Work out the finished part from the listing and answer in its coordinate system (mm). A direction names the side the tool comes from. Round coordinates to 2 decimals unless told otherwise and drop trailing zeros. Write each loop counter-clockwise with the first axis right and the second up, starting at its lowest first coordinate (ties: lowest second). Pieces come first, ordered by that corner, then holes. Notation, with made-up numbers: M 77.25,-8 L 86.25,-8 A18 cw 86.25,6 Z; hole C -28,41.5 d3. An arc over 180 degrees is marked long. One line per item, written item: value. Start each with the question number.
Q1. Consider probe 1 along Y at (x, z) = (24, 0.5); probe 2 along Z at (x, y) = (20, 40.2); probe 3 along Y at (x, z) = (15.5, 2.75). Determine where each line is inside the solid, lowest interval first.
Q2. A tool of negligible diameter and unlimited length cuts with its end or side. For faces 4 (the flat face through (28, 18, 0)), 5 (the cylindrical face through (20.737, 40.918, 6.676)), 6 (the flat face through (3, 42, 10.15)), from which of +Z, -Z, +X, -X, +Y, -Y can it reach the whole face along a straight path? Write none if from no direction.
Q3. Find section B-B (z = -2.5). Write down the section's boundary in (x, y), and give its area (3 significant figures).
Q4. Given pin 1 Ø4.5 at (y, z) = (12, -2.5) entering from -X; pin 2 Ø8 at (x, y) = (18.5, 1.5) entering from -Z; pin 3 Ø1 at (y, z) = (23, 7) entering from -X, each flat-ended and moving along its own axis, determine where each tip first touches the part or whether it passes through.
Q5. Find section C-C (z = 8.5). Write down the section's boundary in (x, y), and give its area (3 significant figures).
Q6. The mould has two halves that part along X. Classify faces 1 (the flat face through (16.584, 42.91, 9.576)), 2 (the flat face through (26.3, 22.44, -1.5)), 3 (the cylindrical face through (9.7, -2.03, 8.95)): released by +X, released by -X, zero draft, split by the parting line, or undercut.
Q7. Find section D-D (x = 20). Write down the section's boundary in (y, z).
Q8. Find section A-A (x = 15.25). Write down the section's boundary in (y, z).
from build123d import *

# Parameters (mm, degrees)
EXTRUDE_1_DEPTH     = 12
SKETCH_2_R          = 4
CUT_EXTRUDE_1_DEPTH = 4
CUT_EXTRUDE_2_DEPTH = 4
SKETCH_4_R          = 1
CUT_EXTRUDE_3_DEPTH = 1.4
CUT_EXTRUDE_4_DEPTH = 4
EXTRUDE_START       = 6
SKETCH_5_W          = 6
SKETCH_5_H          = 5
SKETCH_5_R          = 1
EXTRUDE_2_DEPTH     = 4
EXTRUDE_START_2     = -6
SKETCH_5_2_W        = 6
SKETCH_5_2_H        = 5
SKETCH_5_2_R        = 1
EXTRUDE_3_DEPTH     = 4
FILLET_1_R          = 2


with BuildPart() as part:
    # 草图1 → 凸台-拉伸1 (new body)
    with BuildSketch(Plane.XY):
        Polygon((0, 0), (26, 0), (26, 39.6), (0, 39.6), (0, 43.6), (30, 43.6), (30, -4), (0, -4), align=None)
    extrude(amount=EXTRUDE_1_DEPTH)

    # 草图2 → 切除-拉伸1 (cut)
    with BuildSketch(Plane.XZ.offset(4)):
        with Locations(Location((7, 6, 0), (0, 0, 270))):
            Circle(SKETCH_2_R)
    extrude(amount=-CUT_EXTRUDE_1_DEPTH, mode=Mode.SUBTRACT)

    # 草图3 → 切除-拉伸2 (cut)
    with BuildSketch(Plane(origin=(0, 43.6, 0), x_dir=(1, 0, 0), z_dir=(0, 1, 0))):
        with BuildLine():
            Line((0, -1.85), (0, -10.15))
            Line((0, -10.15), (7, -10.15))
            ThreePointArc((7, -10.15), (11.15, -6), (7, -1.85))
            Line((7, -1.85), (0, -1.85))
        make_face()
    extrude(amount=-CUT_EXTRUDE_2_DEPTH, mode=Mode.SUBTRACT)

    # 草图4 → 切除-拉伸3 (cut)
    with BuildSketch(Plane(origin=(0, 43.6, 0), x_dir=(1, 0, 0), z_dir=(0, 1, 0))):
        with BuildLine():
            ThreePointArc((7.251184211, -1.857608602), (11.15, -6), (7.251184211, -10.142391398))
            Line((7.251184211, -10.142391398), (26.181578947, -8.994499806))
            ThreePointArc((26.181578947, -8.994499806), (29, -6), (26.181578947, -3.005500194))
            Line((26.181578947, -3.005500194), (7.251184211, -1.857608602))
        make_face()
        with Locations(Location((23, -6, 0), (0, 0, 270))):
            Circle(SKETCH_4_R, mode=Mode.SUBTRACT)
        with Locations(Location((20, -6, 0), (0, 0, 270))):
            Circle(SKETCH_4_R, mode=Mode.SUBTRACT)
        with Locations(Location((17, -6, 0), (0, 0, 270))):
            Circle(SKETCH_4_R, mode=Mode.SUBTRACT)
    extrude(amount=-CUT_EXTRUDE_3_DEPTH, mode=Mode.SUBTRACT)

    # 草图4<3> → 切除-拉伸4 (cut)
    with BuildSketch(Plane(origin=(0, 43.6, 0), x_dir=(1, 0, 0), z_dir=(0, 1, 0))):
        with BuildLine():
            ThreePointArc((23, -6), (23.041960108, -6.5), (23.166666667, -6.986013297))
            ThreePointArc((23.166666667, -6.986013297), (23.763762616, -6.645497224), (24, -6))
            Line((24, -6), (23, -6))
        make_face()
        with BuildLine():
            ThreePointArc((22, -6), (22.354502776, -6.763762616), (23.166666667, -6.986013297))
            ThreePointArc((23.166666667, -6.986013297), (23.041960108, -6.5), (23, -6))
            Line((23, -6), (22, -6))
        make_face()
        with BuildLine():
            ThreePointArc((23, -6), (23.041960108, -5.5), (23.166666667, -5.013986703))
            ThreePointArc((23.166666667, -5.013986703), (22.354502776, -5.236237384), (22, -6))
            Line((22, -6), (23, -6))
        make_face()
        with BuildLine():
            ThreePointArc((24, -6), (23.763762616, -5.354502776), (23.166666667, -5.013986703))
            ThreePointArc((23.166666667, -5.013986703), (23.041960108, -5.5), (23, -6))
            Line((23, -6), (24, -6))
        make_face()
        with BuildLine():
            ThreePointArc((21, -6), (20, -5), (19, -6))
            Line((19, -6), (21, -6))
        make_face()
        with BuildLine():
            Line((21, -6), (19, -6))
            ThreePointArc((19, -6), (20, -7), (21, -6))
        make_face()
        with BuildLine():
            ThreePointArc((18, -6), (17, -5), (16, -6))
            Line((16, -6), (18, -6))
        make_face()
        with BuildLine():
            Line((18, -6), (16, -6))
            ThreePointArc((16, -6), (17, -7), (18, -6))
        make_face()
    extrude(amount=-CUT_EXTRUDE_4_DEPTH, mode=Mode.SUBTRACT)

    # 草图5 → 凸台-拉伸2 (add)
    with BuildSketch(Plane(origin=(0, 16.44, 0), x_dir=(1, 0, 0), z_dir=(0, 1, 0)).offset(EXTRUDE_START)):
        with Locations((27, 2.5)):
            Rectangle(SKETCH_5_W, SKETCH_5_H)
        with Locations(Location((27, 2.5, 0), (0, 0, 270))):
            Circle(SKETCH_5_R, mode=Mode.SUBTRACT)
    extrude(amount=EXTRUDE_2_DEPTH)

    # 草图5<2> → 凸台-拉伸3 (add)
    with BuildSketch(Plane(origin=(0, 16.44, 0), x_dir=(1, 0, 0), z_dir=(0, 1, 0)).offset(EXTRUDE_START_2)):
        with Locations((27, 2.5)):
            Rectangle(SKETCH_5_2_W, SKETCH_5_2_H)
        with Locations(Location((27, 2.5, 0), (0, 0, 270))):
            Circle(SKETCH_5_2_R, mode=Mode.SUBTRACT)
    extrude(amount=EXTRUDE_3_DEPTH)

    # 圆角1
    fillet_1_edges = [part.edges().sort_by_distance(p)[0] for p in [
        (26, 12.44, 0),
        (26, 24.44, 0),
    ]]
    fillet(fillet_1_edges, radius=FILLET_1_R - 0.0001)  # a hair under: the kernel refuses the full size


solid = part.part
The answers:
1. probe 1: -4 to 0, 39.6 to 43.6
1. probe 2: 0 to 5, 7 to 12
1. probe 3: -4 to 0, 39.6 to 42.2
2. face 4: -Z, +X, -X
2. face 5: +Y
2. face 6: -X, +Y
3. outline: M 24,10.44 L 26,10.44 L 26,14.44 L 24,14.44 Z; M 24,22.44 L 26,22.44 L 26,26.44 L 24,26.44 Z; M 28,10.44 L 30,10.44 L 30,14.44 L 28,14.44 Z; M 28,22.44 L 30,22.44 L 30,26.44 L 28,26.44 Z
3. area: 32.0 mm2
4. pin 1: x = 24
4. pin 2: z = 0
4. pin 3: x = 26
5. outline: M 0,-4 L 3.88,-4 L 3.88,0 L 0,0 Z; M 10.12,-4 L 30,-4 L 30,43.6 L 27.66,43.6 L 27.66,42.2 L 10.31,42.2 L 10.31,39.6 L 26,39.6 L 26,0 L 10.12,0 Z
5. area: 308 mm2
6. face 1: released by -X
6. face 2: zero draft
6. face 3: undercut
7. outline: M -4,0 L 0,0 L 0,12 L -4,12 Z; M 39.6,0 L 43.6,0 L 43.6,2.63 L 42.2,2.63 L 42.2,5 L 39.6,5 Z; M 39.6,7 L 42.2,7 L 42.2,9.37 L 43.6,9.37 L 43.6,12 L 39.6,12 Z
8. outline: M -4,0 L 0,0 L 0,12 L -4,12 Z; M 39.6,0 L 43.6,0 L 43.6,2.34 L 42.2,2.34 L 42.2,9.66 L 43.6,9.66 L 43.6,12 L 39.6,12 Z
